For this review, take the finished solid that the model builds, in its own axes (mm). A direction names the side the tool comes from. Coordinates: 2 decimals unless noted, no trailing zeros. Loops run counter-clockwise (first coordinate to the right, second up) from the corner with the lowest first, then second, coordinate; pieces in that order, holes last.
1. To check wall thickness, follow probe 1 along Y at (x, z) = (0, 28); probe 2 along Z at (x, y) = (-33, -3); probe 3 along Y at (x, z) = (-5, 12). State the ranges of each line that lie inside material, in increasing order.
2. Take a section at B-B, the plane y = 0. State the section outline as (x, z) points, then the cut area to 4 significant figures.
3. Mouldability with a two-part tool opening along X and no side actions: class faces 5 (the face through (-5, -9, 0)), 6 (the face through (-40, 7, 10)), 7 (the face through (54, -1, 25)) as pulls with the +X half, pulls with the -X half, needs draft (parallel to the pull), parting line crosses it, or undercut.
4. Take a section at A-A, the plane x = 0. State the section outline as (y, z) points, then the cut area to 3 significant figures.
5. Take a section at D-D, the plane x = -35. State the section outline as (y, z) points.
6. Machinability: for faces 1 (the face through (42.4, 18.84, 11.7)), 2 (the face through (35, 0, 47)), 3 (the face through (35, 0, 1)), 4 (the face through (51.97, -8.67, -15.05)), which of the approach directions +Z, -Z, +X, -X, +Y, -Y give a long, thin tool a straight path to every point of the face, cutting with its end or side? Answer none if there is none.
7. Take a section at C-C, the plane z = 8.5. State the section outline as (x, y) points, then the cut area to 3 significant figures.
8. Clearance check with flat-ended pins moving along their axes: P1, Ø0.9, axis at y = 20.5, z = 24.5, coming from the -X side; P2, Ø3, axis at x = 26.5, y = -22.5, coming from the -Z side; P3, Ø23.5, axis at x = -14.5, y = 12.5, coming from the +Z side; P4, Ø12, axis at x = 0, y = 0, coming from the +Z side. State where each tip first meets the part, or that it passes through.
```python
from build123d import *

# Parameters (mm, degrees)
ESQUISSE1_R             = 44
BOSS_EXTRU_1_DEPTH      = 10
ESQUISSE2_R             = 40
BOSS_EXTRU_2_DEPTH      = 28
ESQUISSE3_R             = 44
BOSS_EXTRU_3_DEPTH      = 10
ESQUISSE5_W             = 32.472445712
ESQUISSE5_H             = 94.731646138
ENL_V_MAT_EXTRU_2_DEPTH = 79.587530818
ESQUISSE4_R             = 10
ENL_V_MAT_EXTRU_1_DEPTH = 79.587530818
SKETCH1_R               = 22.5
BOSS_EXTRUDE1_DEPTH     = 15
SKETCH2_R               = 40
BOSS_EXTRUDE2_DEPTH     = 4


with BuildPart() as part:
    # Esquisse1 → Boss.-Extru.1 (new body)
    with BuildSketch(Plane.XY):
        Circle(ESQUISSE1_R)
    extrude(amount=BOSS_EXTRU_1_DEPTH)

    # Esquisse2 → Boss.-Extru.2 (add)
    with BuildSketch(Plane.XY.offset(10)):
        Circle(ESQUISSE2_R)
    extrude(amount=BOSS_EXTRU_2_DEPTH)

    # Esquisse3 → Boss.-Extru.3 (add)
    with BuildSketch(Plane.XY.offset(38)):
        Circle(ESQUISSE3_R)
    extrude(amount=BOSS_EXTRU_3_DEPTH)

    # Esquisse5 → Enlèv. mat.-Extru.2 (cut, through all)
    with BuildSketch(Plane.XY.offset(48)):
        with Locations((51.236222856, -3.296075317)):
            Rectangle(ESQUISSE5_W, ESQUISSE5_H)
    extrude(amount=-ENL_V_MAT_EXTRU_2_DEPTH, mode=Mode.SUBTRACT)

    # Esquisse4 → Enlèv. mat.-Extru.1 (cut, through all)
    with BuildSketch(Plane.XY.offset(48)):
        Circle(ESQUISSE4_R)
    extrude(amount=-ENL_V_MAT_EXTRU_1_DEPTH, mode=Mode.SUBTRACT)

    # Sketch1 → Boss-Extrude1 (add)
    with BuildSketch(Plane(origin=(35, 0, 0), x_dir=(0, 0, -1), z_dir=(1, 0, 0))):
        with Locations(Location((-24, 0, 0), (0, 0, 239.39110234))):
            Circle(SKETCH1_R)
    extrude(amount=BOSS_EXTRUDE1_DEPTH)

    # Sketch2 → Boss-Extrude2 (add)
    with BuildSketch(Plane(origin=(50, 0, 0), x_dir=(0, 0, -1), z_dir=(1, 0, 0))):
        with Locations(Location((-24, 0, 0), (0, 0, 90))):
            Circle(SKETCH2_R)
    extrude(amount=BOSS_EXTRUDE2_DEPTH)


solid = part.part
```
Results list:
1. probe 1: y = -40 to -10, 10 to 40
1. probe 2: z = 0 to 48
1. probe 3: y = -39.69 to -8.66, 8.66 to 39.69
2. outline: (-44, 0) - (-10, 0) - (-10, 48) - (-44, 48) - (-44, 38) - (-40, 38) - (-40, 10) - (-44, 10) - close; (10, 0) - (35, 0) - (35, 1.5) - (50, 1.5) - (50, -16) - (54, -16) - (54, 64) - (50, 64) - (50, 46.5) - (35, 46.5) - (35, 48) - (10, 48) - close
2. area: 3,715 mm2
3. face 5: needs draft
3. face 6: undercut
3. face 7: pulls with the +X half
4. outline: (-44, 0) - (-10, 0) - (-10, 48) - (-44, 48) - (-44, 38) - (-40, 38) - (-40, 10) - (-44, 10) - close; (10, 0) - (44, 0) - (44, 10) - (40, 10) - (40, 38) - (44, 38) - (44, 48) - (10, 48) - close
4. area: 3,040 mm2
5. outline: (-26.66, 0) - (26.66, 0) - (26.66, 10) - (19.36, 10) - (19.36, 38) - (26.66, 38) - (26.66, 48) - (-26.66, 48) - (-26.66, 38) - (-19.36, 38) - (-19.36, 10) - (-26.66, 10) - close
6. face 1: none
6. face 2: +Z
6. face 3: -Z
6. face 4: +X
7. outline: (35, -26.66) - (35, -16.31) - (50, -16.31) - (50, -36.87) - (54, -36.87) - (54, 36.87) - (50, 36.87) - (50, 16.31) - (35, 16.31) - (35, 26.66) arc R44 ccw (long way) to start; hole circle Ø20 at (0, 0)
7. area: 6,230 mm2
8. P1: stops at x = -34.61
8. P2: stops at z = 0
8. P3: stops at z = 48
8. P4: passes through
